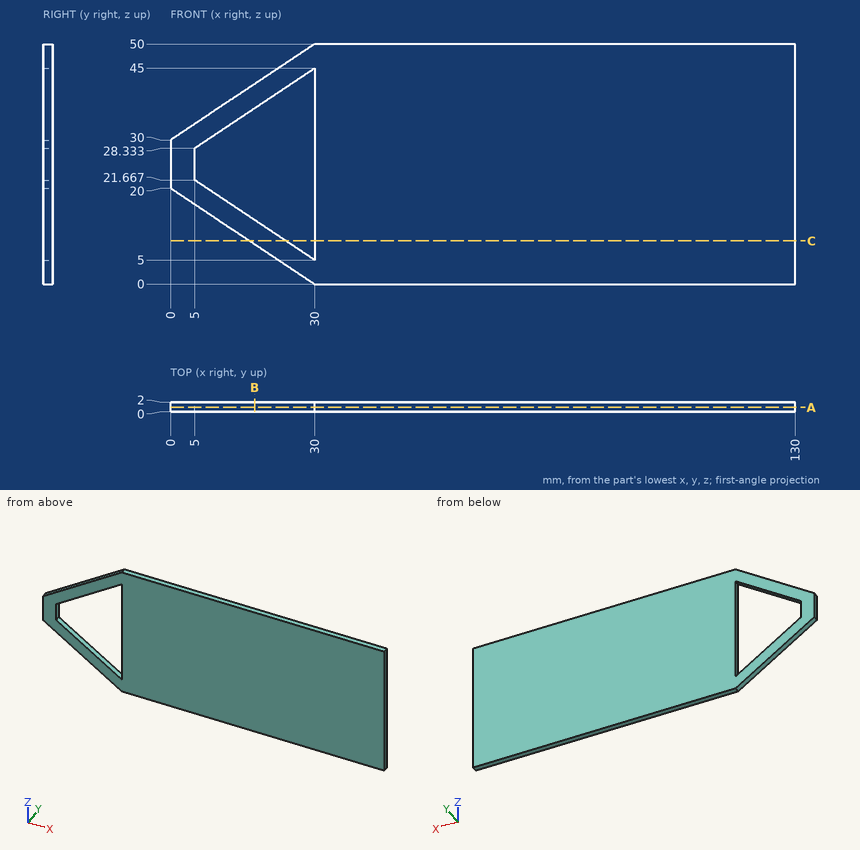
Source: three-view drawing plus pictorial views. Frame: mm from the lowest corner of the part. Round coordinates to 2 decimals unless told otherwise and drop trailing zeros. Order: outer loops, then holes, each group sorted by start corner. A loop starts at its lowest first (then second) coordinate and runs counter-clockwise, first axis right, second up. Notation, with made-up numbers: (27, -4) - (61, -4) arc R19 cw to (61, 30) - close; hole circle Ø9 at (43.25, 73.5). An arc over 180 degrees is marked (long way). Use a Markdown table: item, result.
1. Section C-C on z = 9. Return the cut outline in (x, y).
Evaluation:
| item | result |
|---|---|
| outline | (16.5, 0) - (24, 0) - (24, 2) - (16.5, 2) - close; (30, 0) - (130, 0) - (130, 2) - (30, 2) - close |
2. Material intervals for probe 1 along X at (y, z) = (1.3, 25.5); probe 2 along X at (y, z) = (0.2, 30); probe 3 along Z at (x, y) = (26, 0.65), sorted ascending.
Evaluation:
| item | result |
|---|---|
| probe 1 | 0 to 5, 30 to 130 |
| probe 2 | 0 to 7.5, 30 to 130 |
| probe 3 | 2.67 to 7.67, 42.33 to 47.33 |
3. Section B-B on x = 17.5. Return the cut outline in (y, z), then the cut area to 3 significant figures.
Evaluation:
| item | result |
|---|---|
| outline | (0, 8.33) - (2, 8.33) - (2, 13.33) - (0, 13.33) - close; (0, 36.67) - (2, 36.67) - (2, 41.67) - (0, 41.67) - close |
| area | 20.0 mm^2 |
4. Section A-A on y = 0.9. Return the cut outline in (x, z), then the cut area to 3 significant figures.
Evaluation:
| item | result |
|---|---|
| outline | (0, 20) - (30, 0) - (130, 0) - (130, 50) - (30, 50) - (0, 30) - close; hole (5, 21.67) - (30, 5) - (30, 45) - (5, 28.33) - close |
| area | 5,320 mm^2 |
5. First-contact query: pin 1 (1 mm diameter, centred on y = 1, z = 16, fed in from -X). Flat tip, straight axial feed; report the tip coordinate or a pass-through.
Evaluation:
| item | result |
|---|---|
| pin 1 | x = 5.25 |
